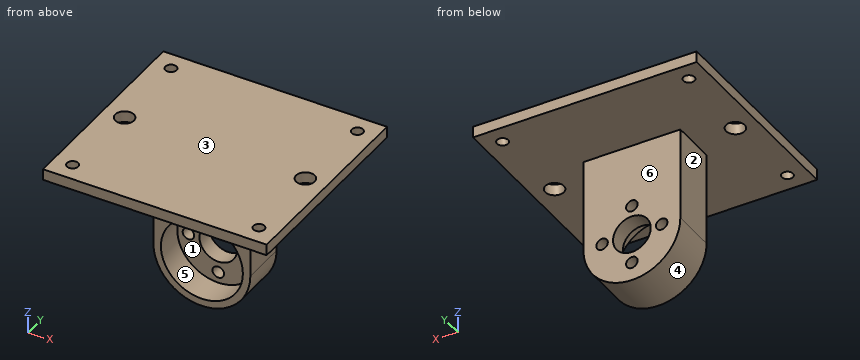
Solid Edge part; units mm, degrees
sketch "Sketch1" plane through (0, 0, 0) normal (0, -1, 0) x (1, 0, 0)
  line L0 (13, 0) -> (13, 25)
  line L1 (13, 25) -> (-13, 25)
  line L2 (-13, 25) -> (-13, 0)
  arc A0 (-13, 0) -> (13, 0) centre (0, 0) ccw
extrude "Protrusion1" add sketch "Sketch1" along normal mid plane 12
sketch "Sketch2" plane through (0, -6, 3.75) normal (0, -1, 0) x (1, 0, 0)
  circle A0 centre (0, -3.75) radius 5.05
extrude "Cutout1" cut sketch "Sketch2" against normal up to next
sketch "Sketch3" plane through (0, -6, 3.75) normal (0, -1, 0) x (1, 0, 0)
  circle A0 centre (0, -3.75) radius 11
extrude "ExtrudedCutout_2" cut sketch "Sketch3" against normal blind 7.5
sketch "Sketch4" plane through (0, 0, 25) normal (0, 0, 1) x (1, 0, 0)
  line L0 (-30, -27.5) -> (30, -27.5)
  line L1 (30, -27.5) -> (30, 27.5)
  line L2 (30, 27.5) -> (-30, 27.5)
  line L3 (-30, 27.5) -> (-30, -27.5)
extrude "ExtrudedProtrusion_3" add sketch "Sketch4" along normal blind 3
sketch "Sketch5" plane through (0, 0, 25) normal (0, 0, -1) x (1, 0, 0)
  circle A0 centre (-24.25, 0) radius 2.5
  circle A1 centre (24.25, 0) radius 2.5
  circle A2 centre (-25, 22.5) radius 1.5
  circle A3 centre (25, 22.5) radius 1.5
  circle A4 centre (25, -22.5) radius 1.5
  circle A5 centre (-25, -22.5) radius 1.5
extrude "Cutout2" cut sketch "Sketch5" against normal up to next
sketch "Sketch6" plane through (0, 1.5, 0) normal (0, -1, 0) x (1, 0, 0)
  circle A0 centre (8, 0) radius 1.55
  circle A1 centre (-8, 0) radius 1.55
  circle A2 centre (0, 8) radius 1.55
  circle A3 centre (0, -8) radius 1.55
extrude "Cutout3" cut sketch "Sketch6" against normal up to next
Verification items for the finished model (mm, model axes). Face numbers are marked on the shaded views. A direction names the side the tool comes from. Coordinates: 2 decimals unless noted, no trailing zeros. Loops run counter-clockwise (first coordinate to the right, second up) from the corner with the lowest first, then second, coordinate; pieces in that order, holes last. Notation, with made-up numbers: (-34.75, -17) -> (0.25, -17) arc R23 cw to (0.25, 0) -> close; hole circle Ø3 at (69, -14). An arc over 180 degrees is marked (long way). Answer in a Markdown table with one row per item.
1) Access from +Z, -Z, +X, -X, +Y, -Y to the whole of each face (thin tool, end or side, straight path). Record for the marked faces 1, 2 and 3.
The answers:
| item | result |
|---|---|
| face 1 | -Y |
| face 2 | -Z, -X, +Y, -Y |
| face 3 | +Z, +X, -X, +Y, -Y |
2) Scan lines: line 1 along X through (y, z) = (0, 27); line 2 along X through (y, z) = (-22, 26); line 3 along Z through (x, y) = (0, 3.35). Record each from-to range of solid material in increasing order. Write a range as from..to.
The answers:
| item | result |
|---|---|
| line 1 | x = -30..-26.75, -21.75..21.75, 26.75..30 |
| line 2 | x = -30..-26.41, -23.59..23.59, 26.41..30 |
| line 3 | z = -13..-9.55, -6.45..-5.05, 5.05..6.45, 9.55..28 |
3) Depth check by flat-ended pin: P1, Ø6, axis at x = -14.5, z = -7, coming from the -Y side; P2, Ø13, axis at x = 1, z = 7, coming from the -Y side; P3, Ø2, axis at y = -0.5, z = -4.5, coming from the +X side; P4, Ø5, axis at x = 0, z = -8, coming from the +Y side. Enter the tip coordinate at first touch or a pass-through.
The answers:
| item | result |
|---|---|
| P1 | passes through |
| P2 | stops at y = -6 |
| P3 | stops at x = 12.52 |
| P4 | stops at y = 6 |
4) Section check D-D (x = 8). Record the cut outline in (y, z).
The answers:
| item | result |
|---|---|
| outline | (-27.5, 25) -> (-6, 25) -> (-6, 7.55) -> (1.5, 7.55) -> (1.5, 1.55) -> (6, 1.55) -> (6, 25) -> (27.5, 25) -> (27.5, 28) -> (-27.5, 28) -> close; (-6, -10.25) -> (6, -10.25) -> (6, -1.55) -> (1.5, -1.55) -> (1.5, -7.55) -> (-6, -7.55) -> close |
5) Draft check along X on the marked faces 4, 5 and 6. Enter one of: released by +X, released by -X, zero draft, split by the parting line, or undercut.
The answers:
| item | result |
|---|---|
| face 4 | split by the parting line |
| face 5 | undercut |
| face 6 | zero draft |
6) Section check C-C (z = 4). Record the cut outline in (x, y), and give its area (3 significant figures).
The answers:
| item | result |
|---|---|
| outline | (-13, -6) -> (-10.25, -6) -> (-10.25, 1.5) -> (-3.08, 1.5) -> (-3.08, 6) -> (-13, 6) -> close; (3.08, 1.5) -> (10.25, 1.5) -> (10.25, -6) -> (13, -6) -> (13, 6) -> (3.08, 6) -> close |
| area | 131 mm2 |
7) Section check A-A (x = 0). Record the cut outline in (y, z), and give its area (3 significant figures).
The answers:
| item | result |
|---|---|
| outline | (-27.5, 25) -> (-6, 25) -> (-6, 11) -> (1.5, 11) -> (1.5, 9.55) -> (6, 9.55) -> (6, 25) -> (27.5, 25) -> (27.5, 28) -> (-27.5, 28) -> close; (-6, -13) -> (6, -13) -> (6, -9.55) -> (1.5, -9.55) -> (1.5, -11) -> (-6, -11) -> close; (1.5, -6.45) -> (6, -6.45) -> (6, -5.05) -> (1.5, -5.05) -> close; (1.5, 5.05) -> (6, 5.05) -> (6, 6.45) -> (1.5, 6.45) -> close |
| area | 383 mm2 |
8) Section check B-B (y = -22.5). Record the cut outline in (x, z), and give its area (3 significant figures).
The answers:
| item | result |
|---|---|
| outline | (-30, 25) -> (-26.5, 25) -> (-26.5, 28) -> (-30, 28) -> close; (-23.5, 25) -> (23.5, 25) -> (23.5, 28) -> (-23.5, 28) -> close; (26.5, 25) -> (30, 25) -> (30, 28) -> (26.5, 28) -> close |
| area | 162 mm2 |
